Study the drawing (mm; zero at the part's minimum x, y, z) and answer. Round coordinates to 2 decimals unless told otherwise and drop trailing zeros. Loops run counter-clockwise (first coordinate to the right, second up) from the corner with the lowest first, then second, coordinate; pieces in that order, holes last. Notation, with made-up numbers: M 14.5,7 L 37.5,7 A10 ccw 37.5,12 Z; hole C 45.5,76 d7. An arc over 180 degrees is marked long. Put each result on its own line as item: value. Start each with the question number.
(1) Section B-B, the plane x = 350 is taken. Determine the outline of the cut face in (y, z), then the cut area to 3 significant figures.
(2) Section C-C, the plane z = 3.5 is taken. Determine the outline of the cut face in (x, y), then the cut area to 3 significant figures.
(3) Straight lines are drawn through the part: line 1 (X direction, y = 240, z = 7); line 2 (Y direction, x = 350, z = 5); line 3 (X direction, y = 106.5, z = 5.5). For each, find the intervals that lie inside material, in ascending order.
(4) Section A-A, the plane y = 240 is taken. Determine the outline of the cut face in (x, z).
(5) A flat-ended cylindrical pin translates along its axis: P1, Ø5, axis at x = 376, z = 5.5, coming from the -Y side. Find the tip coordinate at first contact, or state that the pin passes through.
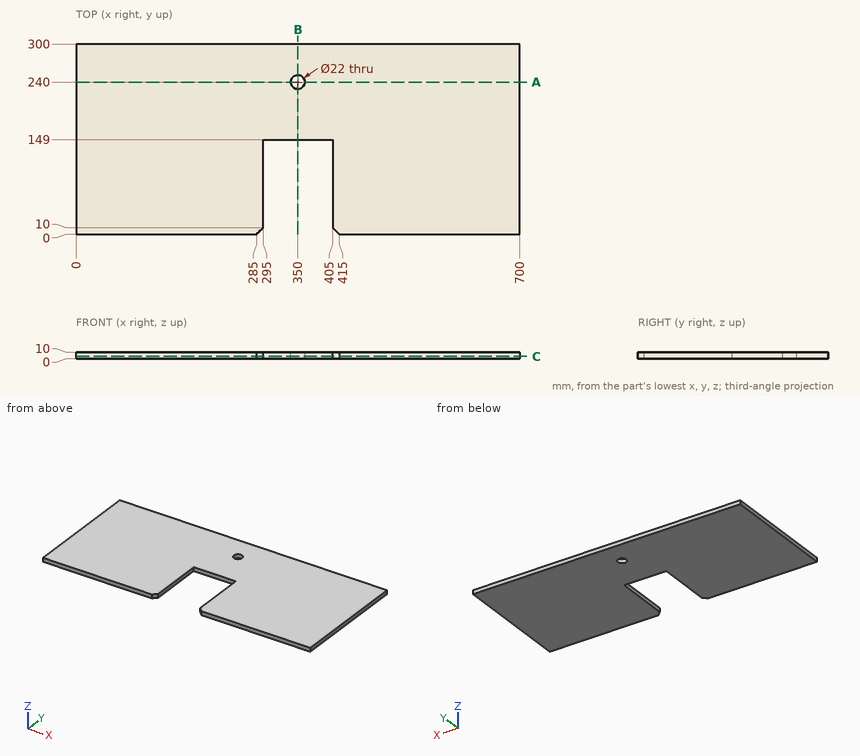
Recorded:
1. outline: M 149,0 L 229,0 L 229,10 L 149,10 Z; M 251,0 L 300,0 L 300,10 L 251,10 Z
1. area: 1,290 mm²
2. outline: M 0,0 L 285,0 L 295,10 L 295,149 L 405,149 L 405,10 L 415,0 L 700,0 L 700,300 L 0,300 Z; hole C 350,240 d22
2. area: 193,000 mm²
3. line 1: x = 0 to 339, 361 to 700
3. line 2: y = 149 to 229, 251 to 300
3. line 3: x = 0 to 295, 405 to 700
4. outline: M 0,0 L 339,0 L 339,10 L 0,10 Z; M 361,0 L 700,0 L 700,10 L 361,10 Z
5. P1: stops at y = 149
